Can you work these out from the model? Positions are in its coordinate system, mm. Coordinates: 2 decimals unless noted, no trailing zeros. Order: outer loops, then holes, each group sorted by start corner. A loop starts at its lowest first (then second) coordinate and runs counter-clockwise, first axis right, second up. Notation, with made-up numbers: (81.5, 39) -> (101.5, 39) arc R17 ccw to (101.5, 67) -> close; hole circle Ø4 at (53, 13). An arc over 180 degrees is marked (long way). Answer in a Markdown table with one row per item.
Autodesk Inventor part; units mm, degrees
ref_plane "YZ Plane" through (0, 0, 0) normal (1, 0, 0) x (0, 1, 0)
ref_plane "XZ Plane" through (0, 0, 0) normal (0, 1, 0) x (-1, 0, 0)
ref_plane "XY Plane" through (0, 0, 0) normal (0, 0, 1) x (1, 0, 0)
sketch "Sketch1" plane through (0, 0, 0) normal (0, 1, 0) x (-1, 0, 0)
  circle A0 centre (0, 25) radius 5
  arc A1 (10, 25) -> (-10, 25) centre (0, 25) ccw
  arc A2 (-10, -25) -> (10, -25) centre (0, -25) ccw
  circle A3 centre (0, -25) radius 5
  line L0 (10, 25) -> (10, -25)
  line L1 (-10, -25) -> (-10, 25)
  line L2 (10, 25) -> (10, 35)
  line L3 (-10, 25) -> (-10, 35)
  line L4 (-10, 35) -> (10, 35)
  line L5 (-10, -25) -> (-10, -35)
  line L6 (-10, -35) -> (10, -35)
  line L7 (10, -35) -> (10, -25)
  point P0 (0, 0)
  point P1 (10, 0)
  point P2 (0, -35)
  point P3 (0, 35)
  dimension "d0" = 50
  dimension "d1" = 10
  dimension "d2" = 20
extrude "Extrusion1" add sketch "Sketch1" along normal mid plane 5 contours L0 A2 L1 A1
extrude "Extrusion2" [suppressed]
chamfer "Chamfer1" distance 0.5 angle 45 8 edges at (-10, -2.5, 0) (0, -2.5, -35) (0, -2.5, 35) (10, -2.5, 0) (-10, 2.5, 0) (0, 2.5, 35) (10, 2.5, 0) (0, 2.5, -35)
properties part number "LINK" material "Aluminium 6082 T6"
(1) Suppose I cut it at A-A (z = -22). Please give me the cut outline in (x, y).
Response values:
| item | result |
|---|---|
| outline | (-10, -2) -> (-9.5, -2.5) -> (-4, -2.5) -> (-4, 2.5) -> (-9.5, 2.5) -> (-10, 2) -> close; (4, -2.5) -> (9.5, -2.5) -> (10, -2) -> (10, 2) -> (9.5, 2.5) -> (4, 2.5) -> close |
(2) I need wall thicknesses on line 1 (Z direction, x = 0, y = -0.4); line 2 (Z direction, x = 3.25, y = -1.45); line 3 (X direction, y = -2.1, z = -25.5). Which ranges of each line are inside material? Lowest first, please. Write a range as [from, to].
Response values:
| item | result |
|---|---|
| line 1 | [-35, -30], [-20, 20], [30, 35] |
| line 2 | [-34.46, -28.8], [-21.2, 21.2], [28.8, 34.46] |
| line 3 | [-9.89, -4.97], [4.97, 9.89] |
(3) Will these pins go through, and if not, where does the flat tip stop? pin 1 Ø9 at (x, z) = (0, 25) entering from +Y; pin 2 Ø1.5 at (x, y) = (1.5, 1.5) entering from +Z.
Response values:
| item | result |
|---|---|
| pin 1 | through |
| pin 2 | z = 34.97 |
(4) Suppose I cut it at B-B (x = 0). Please give me the cut outline in (y, z), and give its area (4 significant figures).
Response values:
| item | result |
|---|---|
| outline | (-2.5, -34.5) -> (-2, -35) -> (2, -35) -> (2.5, -34.5) -> (2.5, -30) -> (-2.5, -30) -> close; (-2.5, -20) -> (2.5, -20) -> (2.5, 20) -> (-2.5, 20) -> close; (-2.5, 30) -> (2.5, 30) -> (2.5, 34.5) -> (2, 35) -> (-2, 35) -> (-2.5, 34.5) -> close |
| area | 249.5 mm2 |
